Autodesk Inventor part; units mm, degrees
ref_plane "YZ Plane" through (0, 0, 0) normal (1, 0, 0) x (0, 1, 0)
ref_plane "XZ Plane" through (0, 0, 0) normal (0, 1, 0) x (-1, 0, 0)
ref_plane "XY Plane" through (0, 0, 0) normal (0, 0, 1) x (1, 0, 0)
sketch "Sketch1" plane through (0, 0, 0) normal (0, 0, 1) x (1, 0, 0)
  line L0 (-7.3323, 0) -> (-3.6662, 6.35)
  line L1 (-3.6662, 6.35) -> (3.6662, 6.35)
  line L2 (3.6662, 6.35) -> (7.3323, 0)
  line L3 (7.3323, 0) -> (3.6662, -6.35)
  line L4 (3.6662, -6.35) -> (-3.6662, -6.35)
  line L5 (-3.6662, -6.35) -> (-7.3323, 0)
  point P0 (0, 0)
  point P1 (0, 0)
  dimension "d0" = 12.7
extrude "Extrusion1" add sketch "Sketch1" along normal mid plane 45.512
sketch "Sketch2" plane through (0, 0, 22.756) normal (0, 0, 1) x (1, 0, 0)
  point P0 (0, 0)
hole "Hole1" at (0, 0, 22.756) direction (0, 0, -1) diameter 3.683 end through all
mirror "Mirror1" about plane through (0, 0, 0) normal (0, 0, 1) of "Hole1"
properties part number "PULLY_HEX_SHAFT_INTAKE" material "Aluminum, 6061-T6"
Work out the finished part from the listing and answer in its coordinate system (mm). Round coordinates to 2 decimals unless told otherwise and drop trailing zeros. Loops run counter-clockwise (first coordinate to the right, second up) from the corner with the lowest first, then second, coordinate; pieces in that order, holes last. Notation, with made-up numbers: M -17.75,2 L 16.25,2 A32 cw 16.25,38 Z; hole C 79.25,8.5 d2. An arc over 180 degrees is marked long. One line per question, with ' | ' between items. Start each with the question number.
(1) A flat-ended cylindrical pin translates along its axis: pin 1 Ø1 at (y, z) = (-4.5, -0.5) entering from +X. Find the tip coordinate at first contact, or state that the pin passes through.
(2) Find the intervals of material crossed by line 1 (Y direction, x = 0, z = 11); line 2 (X direction, y = 0, z = 0.5); line 3 (Y direction, x = -1, z = 0), in increasing order.
(3) A cutting plane is placed at A-A on x = 0. Write down the section's boundary in (y, z).
(4) A cutting plane is placed at B-B on z = 7. Write down the section's boundary in (x, y).
(5) For a pull along X with two mould halves and no side action, classify faces 1 (the face through (-5.474, -3.219, -0.319)), 2 (the face through (5.474, 3.219, -0.319)), 3 (the face through (1.634, -0.85, -0.319)) as released by +X, released by -X, zero draft, split by the parting line, or undercut.
(6) A cutting plane is placed at D-D on y = -3. Write down the section's boundary in (x, z), plus the area to 3 significant figures.
(7) A cutting plane is placed at C-C on x = -4.5. Write down the section's boundary in (y, z).
Geometry check:
1) pin 1: stops at x = 5.02
2) line 1: y = -6.35 to -1.84, 1.84 to 6.35 | line 2: x = -7.33 to -1.84, 1.84 to 7.33 | line 3: y = -6.35 to -1.55, 1.55 to 6.35
3) outline: M -6.35,-22.76 L -1.84,-22.76 L -1.84,22.76 L -6.35,22.76 Z; M 1.84,-22.76 L 6.35,-22.76 L 6.35,22.76 L 1.84,22.76 Z
4) outline: M -7.33,0 L -3.67,-6.35 L 3.67,-6.35 L 7.33,0 L 3.67,6.35 L -3.67,6.35 Z; hole C 0,0 d3.68
5) face 1: released by -X | face 2: released by +X | face 3: undercut
6) outline: M -5.6,-22.76 L 5.6,-22.76 L 5.6,22.76 L -5.6,22.76 Z | area: 510 mm²
7) outline: M -4.91,-22.76 L 4.91,-22.76 L 4.91,22.76 L -4.91,22.76 Z
